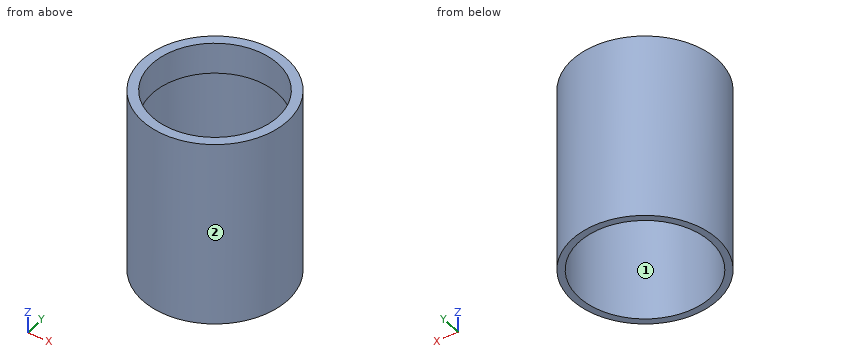
Autodesk Inventor part; units mm, degrees
ref_plane "YZ Plane" through (0, 0, 0) normal (1, 0, 0) x (0, 1, 0)
ref_plane "XZ Plane" through (0, 0, 0) normal (0, 1, 0) x (-1, 0, 0)
ref_plane "XY Plane" through (0, 0, 0) normal (0, 0, 1) x (1, 0, 0)
sketch "Sketch1" plane through (0, 0, 0) normal (0, 0, 1) x (1, 0, 0)
  circle A0 centre (-13.5074, 0) radius 22.098
  point P0 (0, 0)
  dimension "d0" = 44.196
extrude "Extrusion1" add sketch "Sketch1" along normal blind 57.15
sketch "Sketch2" plane through (-13.5074, 0, 57.15) normal (0, 0, 1) x (1, 0, 0)
  circle A0 centre (0, 0) radius 22.098
  point P0 (13.5074, 0)
hole "Hole1" at (-13.5074, 0, 57.15) direction (0, 0, -1) diameter 38.3032 depth 10.16 tip angle 118
sketch "Sketch3" plane through (-13.5074, 0, 0) normal (0, 0, -1) x (-1, 0, 0)
  circle A0 centre (0, 0) radius 22.098
  circle A1 centre (0, 0) radius 20.0279
  point P0 (-13.5074, 0)
  dimension "d10" = 40.0558
extrude "Extrusion2" cut sketch "Sketch3" against normal blind 47.625 contours A1
properties part number "JF-AT-JC0005" material "Acrylic, Clear"
Input: part model. Units: mm. Frame: model coordinates. Face numbers are marked on the shaded views. Give positions to 0.01 mm unless a question says otherwise; leave off trailing zeros. Write each loop counter-clockwise with the first axis right and the second up, starting at its lowest first coordinate (ties: lowest second). Pieces come first, ordered by that corner, then holes.
Q1. Section B-B, the plane x = 0. Output: boundary loops of the cut face in (y, z) (3 decimals), plus the area to 3 significant figures.
Q2. Section C-C, the plane z = 39. Output: boundary loops of the cut face in (x, y), plus the area to 3 significant figures.
Q3. First-contact query: P1, Ø3, axis at y = 13.5, z = 6.5, coming from the +X side; P2, Ø1.5, axis at y = 11, z = 8.5, coming from the -X side; P3, Ø3, axis at x = -22, z = 28.5, coming from the +Y side; P4, Ø12, axis at y = 1, z = 20, coming from the -X side. Flat tips, straight axial feed; report the tip coordinate or a pass-through.
Q4. Material intervals for probe 1 along Y at (x, z) = (-13.5, 24); probe 2 along Z at (x, y) = (-8.5, 19) (3 decimals); probe 3 along Y at (x, z) = (4, 33), sorted ascending.
Q5. Pull-direction query (X, two-part tool) for the marked faces 1 and 2; classes: pulls with the +X half, pulls with the -X half, needs draft (parallel to the pull), parting line crosses it, or undercut.
Filled in:
1. outline: (-17.489, 0) - (-14.787, 0) - (-14.787, 47.625) - (-13.577, 47.625) - (-13.577, 57.15) - (-17.489, 57.15) - close; (13.577, 47.625) - (14.787, 47.625) - (14.787, 0) - (17.489, 0) - (17.489, 57.15) - (13.577, 57.15) - close
1. area: 332 mm2
2. outline: circle Ø44.2 at (-13.51, 0); hole circle Ø40.06 at (-13.51, 0)
2. area: 274 mm2
3. P1: stops at x = 5.05
3. P2: stops at x = -33.08
3. P3: stops at y = 20.96
3. P4: stops at x = -35.61
4. probe 1: y = -22.1 to -20.03, 20.03 to 22.1
4. probe 2: z = 47.625 to 57.15
4. probe 3: y = -13.48 to -9.73, 9.73 to 13.48
5. face 1: undercut
5. face 2: parting line crosses it
